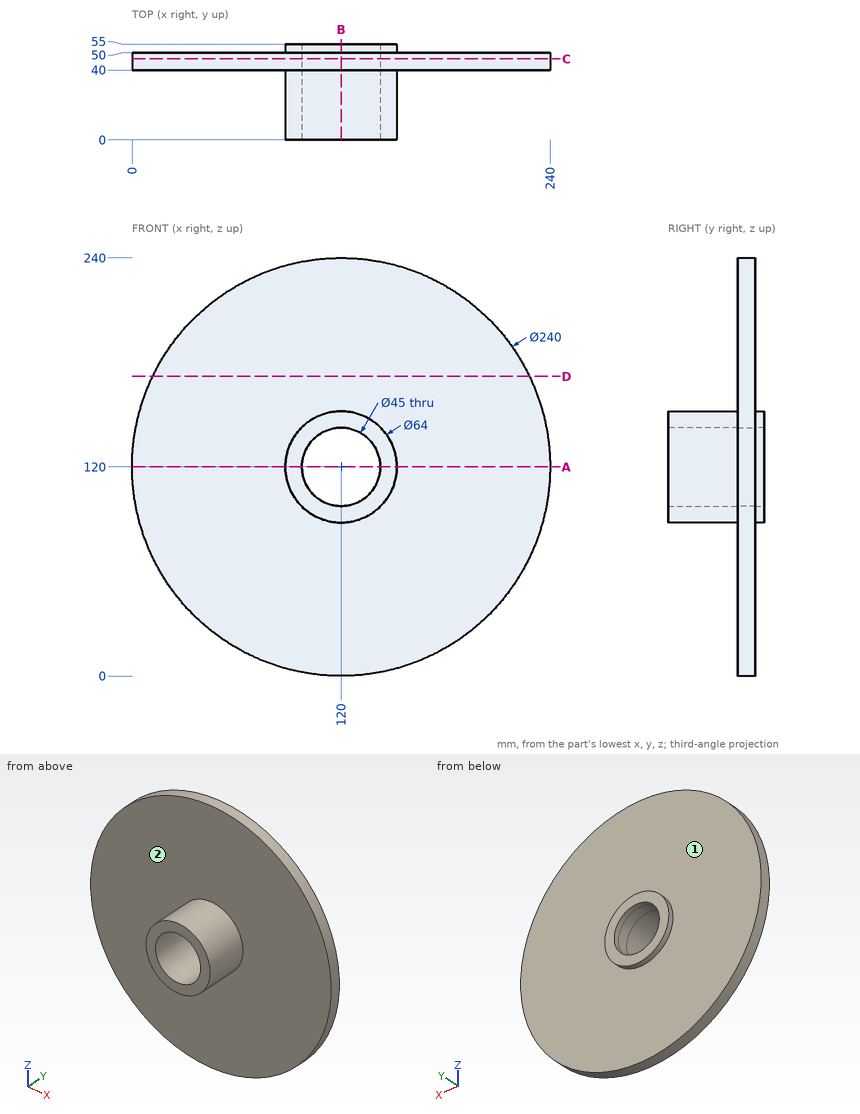
Job drawing, mm, ordinate dimensions from the low corner. One solid piece. A direction names the side the tool comes from. Round coordinates to 2 decimals unless told otherwise and drop trailing zeros. Loops run counter-clockwise (first coordinate to the right, second up) from the corner with the lowest first, then second, coordinate; pieces in that order, holes last. Notation, with made-up numbers: (-11.75, 23) -> (24.25, 23) arc R7 ccw to (24.25, 28) -> close; hole circle Ø5 at (30.25, 10.25). An arc over 180 degrees is marked (long way). One line per item, written item: value. Start each with the question number.
Q1. Cut at C-C on y = 46.5. List the corners of the cut face in (x, z).
Q2. 3-axis set-ups, long thin cutter, end or side, ignore diameter. For the marked faces 1 and 2: which of +Z, -Z, +X, -X, +Y, -Y reach the whole face in a straight line?
Q3. Drop flat-ended pins along their axis: pin 1 Ø8 at (x, y) = (172, 35.5) entering from -Z; pin 2 Ø10 at (x, z) = (170.5, 190.5) entering from -Y; pin 3 Ø1 at (x, z) = (132.5, 159.5) entering from +Y; pin 4 Ø12 at (x, y) = (114.5, 12.5) entering from +Z. Give the stop position or say it passes through.
Q4. Probe line 1 along X through (y, z) = (17, 120); line 2 along Y through (x, z) = (205, 54). List the from-to ranges inside material, lowest first.
Q5. Cut at A-A on z = 120. List the corners of the cut face in (x, y), plus the area to 4 significant figures.
Q6. Cut at B-B on x = 120. List the corners of the cut face in (y, z).
Q7. Cut at D-D on z = 172. List the corners of the cut face in (x, y).
Computed:
1. outline: circle Ø240 at (120, 120); hole circle Ø45 at (120, 120)
2. face 1: +Y
2. face 2: -Y
3. pin 1: through
3. pin 2: y = 40
3. pin 3: y = 50
3. pin 4: z = 152
4. line 1: 88 to 97.5, 142.5 to 152
4. line 2: 40 to 50
5. outline: (0, 40) -> (88, 40) -> (88, 0) -> (97.5, 0) -> (97.5, 55) -> (88, 55) -> (88, 50) -> (0, 50) -> close; (142.5, 0) -> (152, 0) -> (152, 40) -> (240, 40) -> (240, 50) -> (152, 50) -> (152, 55) -> (142.5, 55) -> close
5. area: 2,805 mm²
6. outline: (0, 88) -> (40, 88) -> (40, 0) -> (50, 0) -> (50, 88) -> (55, 88) -> (55, 97.5) -> (0, 97.5) -> close; (0, 142.5) -> (55, 142.5) -> (55, 152) -> (50, 152) -> (50, 240) -> (40, 240) -> (40, 152) -> (0, 152) -> close
7. outline: (11.85, 40) -> (228.15, 40) -> (228.15, 50) -> (11.85, 50) -> close
